```python
from build123d import *

# Parameters (mm, degrees)
F1_DEPTH = 6.35
F3_DEPTH = 6.35


with BuildPart() as f1:
    # F0 (on Top) → F1 (new body)
    with BuildSketch(Plane.XY):
        Polygon((-116.137687, 0), (-116.137687, -61.976), (-68.512687, -61.976), (-68.512687, -55.626), (-62.162687, -55.626), (-62.162687, -49.276), (-36.762687, -49.276), (-36.762687, -55.626), (-30.412687, -55.626), (-30.412687, -61.976), (185.487313, -61.976), (185.487313, -55.626), (191.837313, -55.626), (191.837313, -49.276), (217.237313, -49.276), (217.237313, -55.626), (223.587313, -55.626), (223.587313, -61.976), (271.212313, -61.976), (271.212313, 0), align=None)
    extrude(amount=F1_DEPTH)

    # F2 (on face) → F3 (join)
    with BuildSketch(Plane.XY.offset(6.35)):
        Polygon((290.262313, 0), (271.212313, 0), (271.212313, -9.525), (277.562313, -9.525), (277.562313, -19.05), (290.262313, -19.05), align=None)
        Polygon((-116.137687, -9.525), (-116.137687, 0), (-135.187687, 0), (-135.187687, -19.05), (-122.487687, -19.05), (-122.487687, -9.525), align=None)
    extrude(amount=-F3_DEPTH)


solid = f1.part
```
Can you work these out from the model? Positions are in its coordinate system, mm. Round coordinates to 2 decimals unless told otherwise and drop trailing zeros. Loops run counter-clockwise (first coordinate to the right, second up) from the corner with the lowest first, then second, coordinate; pieces in that order, holes last. Notation, with made-up numbers: (-14.5, 46) -> (-5.5, 46) arc R23 ccw to (-5.5, 73) -> close; hole circle Ø2 at (51, -16). An arc over 180 degrees is marked (long way). Answer in a Markdown table with one row per item.
Item 1: Will these pins go through, and if not, where does the flat tip stop? P1, Ø1.9, axis at y = -29.5, z = 3, coming from the +X side; P2, Ø2, axis at x = 139, z = 2, coming from the +Y side; P3, Ø1.9, axis at y = -53, z = 2.5, coming from the -X side; P4, Ø1.9, axis at x = 190, z = 3, coming from the -Y side.
Answer block:
| item | result |
|---|---|
| P1 | x = 271.21 |
| P2 | y = 0 |
| P3 | x = -116.14 |
| P4 | y = -55.63 |
Item 2: Suppose I cut it at A-A, the plane z = 1.5. List the corners of the cut face in (x, y) for me (3 decimals), plus the area to 3 significant figures.
Answer block:
| item | result |
|---|---|
| outline | (-135.188, -19.05) -> (-122.488, -19.05) -> (-122.488, -9.525) -> (-116.138, -9.525) -> (-116.138, -61.976) -> (-68.513, -61.976) -> (-68.513, -55.626) -> (-62.163, -55.626) -> (-62.163, -49.276) -> (-36.763, -49.276) -> (-36.763, -55.626) -> (-30.413, -55.626) -> (-30.413, -61.976) -> (185.487, -61.976) -> (185.487, -55.626) -> (191.837, -55.626) -> (191.837, -49.276) -> (217.237, -49.276) -> (217.237, -55.626) -> (223.587, -55.626) -> (223.587, -61.976) -> (271.212, -61.976) -> (271.212, -9.525) -> (277.562, -9.525) -> (277.562, -19.05) -> (290.262, -19.05) -> (290.262, 0) -> (-135.188, 0) -> close |
| area | 23,800 mm² |
Item 3: If I drill on probe 1 along X at (y, z) = (-53, 3); probe 2 along X at (y, z) = (-18, 2.5); probe 3 along X at (y, z) = (-32.5, 4.75), over which ranges is the centre line in solid material (lowest first)?
Answer block:
| item | result |
|---|---|
| probe 1 | -116.14 to -62.16, -36.76 to 191.84, 217.24 to 271.21 |
| probe 2 | -135.19 to -122.49, -116.14 to 271.21, 277.56 to 290.26 |
| probe 3 | -116.14 to 271.21 |
Item 4: Suppose I cut it at B-B, the plane x = 203. List the corners of the cut face in (y, z) for me.
Answer block:
| item | result |
|---|---|
| outline | (-49.28, 0) -> (0, 0) -> (0, 6.35) -> (-49.28, 6.35) -> close |
Item 5: Suppose I cut it at C-C, the plane y = -30.5. List the corners of the cut face in (x, z) for me.
Answer block:
| item | result |
|---|---|
| outline | (-116.14, 0) -> (271.21, 0) -> (271.21, 6.35) -> (-116.14, 6.35) -> close |
